from build123d import *

# Parameters (mm, degrees)
SKETCH1_W           = 10
SKETCH1_H           = 2.5
BOSS_EXTRUDE1_DEPTH = 7
SKETCH2_W           = 9.8
SKETCH2_H           = 2.3
BOSS_EXTRUDE2_DEPTH = 0.1
SKETCH3_W           = 1.487009638
SKETCH3_H           = 2.3
BOSS_EXTRUDE3_DEPTH = 0.5


with BuildPart() as part:
    # Sketch1 → Boss-Extrude1 (new body)
    with BuildSketch(Plane(origin=(0, 0, 0), x_dir=(1, 0, 0), z_dir=(0, 1, 0))):
        Rectangle(SKETCH1_W, SKETCH1_H)
    extrude(amount=BOSS_EXTRUDE1_DEPTH)

    # Sketch2 → Boss-Extrude2 (add)
    with BuildSketch(Plane(origin=(0, 7, 0), x_dir=(1, 0, 0), z_dir=(0, 1, 0))):
        Rectangle(SKETCH2_W, SKETCH2_H)
    extrude(amount=BOSS_EXTRUDE2_DEPTH)

    # Sketch3 → Boss-Extrude3 (add)
    with BuildSketch(Plane(origin=(0, 7.1, 0), x_dir=(1, 0, 0), z_dir=(0, 1, 0))):
        with Locations((-2.868353266, 0)):
            Rectangle(SKETCH3_W, SKETCH3_H)
    extrude(amount=BOSS_EXTRUDE3_DEPTH)


solid = part.part
Geometry: final body of the model. Coordinates: model frame, mm. A direction names the side the tool comes from. Give positions to 0.01 mm unless a question says otherwise; leave off trailing zeros. Order: outer loops, then holes, each group sorted by start corner. A loop starts at its lowest first (then second) coordinate and runs counter-clockwise, first axis right, second up. Notation, with made-up numbers: (46.25, -14) -> (80.25, -14) arc R27 ccw to (80.25, 13) -> close; hole circle Ø3 at (47, -40). An arc over 180 degrees is marked (long way). Answer as a JSON object with one key per item and string values.
Q1. Section A-A (z = 0.95). Output: boundary loops of the cut face in (x, y), plus the area to 3 significant figures.
Entries:
{"outline": "(-5, 0) -> (5, 0) -> (5, 7) -> (4.9, 7) -> (4.9, 7.1) -> (-2.12, 7.1) -> (-2.12, 7.6) -> (-3.61, 7.6) -> (-3.61, 7.1) -> (-4.9, 7.1) -> (-4.9, 7) -> (-5, 7) -> close", "area": "71.7 mm^2"}
Q2. First-contact query: pin 1 (1 mm diameter, centred on x = -2.5, z = 1, fed in from -Y); pin 2 (0.7 mm diameter, centred on x = 0, y = 7.5, fed in from +Z); pin 3 (0.6 mm diameter, centred on x = -4.5, z = 0, fed in from +Y); pin 4 (0.6 mm diameter, centred on y = 7.5, z = 0.5, fed in from -X). Flat tips, straight axial feed; report the tip coordinate or a pass-through.
Entries:
{"pin 1": "stops at y = 0", "pin 2": "passes through", "pin 3": "stops at y = 7.1", "pin 4": "stops at x = -3.61"}
Q3. Material intervals for probe 1 along Y at (x, z) = (2.25, 1); probe 2 along X at (y, z) = (7.25, 0.2), sorted ascending.
Entries:
{"probe 1": "y = 0 to 7.1", "probe 2": "x = -3.61 to -2.12"}
Q4. Access query for faces 1 (the flat face through (-4, 7.1, 0)), 2 (the flat face through (0, 0, 0)), 3 (the flat face through (1, 7.1, 0)). Directions: +Z, -Z, +X, -X, +Y, -Y. A direction counts if a zero-diameter tool reaches every point of the face in a straight line with its end or side. Return the directions, or none.
Entries:
{"face 1": "+Z, -Z, -X, +Y", "face 2": "+Z, -Z, +X, -X, -Y", "face 3": "+Z, -Z, +X, +Y"}
Q5. Section B-B (x = -0.5). Output: boundary loops of the cut face in (y, z).
Entries:
{"outline": "(0, -1.25) -> (7, -1.25) -> (7, -1.15) -> (7.1, -1.15) -> (7.1, 1.15) -> (7, 1.15) -> (7, 1.25) -> (0, 1.25) -> close"}
